```python
from build123d import *

# Parameters (mm, degrees)
F0_R             = 21
F1_DEPTH         = 7
F3_DEPTH         = 3
F4_R             = 3.35
F5_DEPTH         = 2
F6_R             = 0.5
F7_DEPTH         = 3.4
F8_R             = 5
F9_DEPTH         = 5.5
F13_COPIES_COUNT = 4


# Not quite as in the source:
# - a pattern or mirror of a feature is missing from the dataset's text; its kind, count and spacing are read off the source's solid


with BuildPart() as f1:
    # F0 (on Top) → F1 (new body)
    with BuildSketch(Plane.XY):
        Circle(F0_R)
    extrude(amount=F1_DEPTH)

    # F2 (on face) → F3 (cut)
    with BuildSketch(Plane.XY.offset(7)):
        with BuildLine():
            Line((-2.5, 16.8585155142), (-4.3, 4.4317744753))
            ThreePointArc((-4.3, 4.4317744753), (-6.175, 0), (-4.3, -4.4317744753))
            Line((-4.3, -4.4317744753), (-2.5, -16.8585155142))
            ThreePointArc((-2.5, -16.8585155142), (-1.6521982913, -18.3987898667), (0, -19))
            ThreePointArc((0, -19), (1.6521982913, -18.3987898667), (2.5, -16.8585155142))
            Line((2.5, -16.8585155142), (4.3, -4.4317744753))
            ThreePointArc((4.3, -4.4317744753), (6.175, 0), (4.3, 4.4317744753))
            Line((4.3, 4.4317744753), (2.5, 16.8585155142))
            ThreePointArc((2.5, 16.8585155142), (1.6521982913, 18.3987898667), (0, 19))
            ThreePointArc((0, 19), (-1.6521982913, 18.3987898667), (-2.5, 16.8585155142))
        make_face()
    extrude(amount=-F3_DEPTH, mode=Mode.SUBTRACT)

    # F4 (on face) → F5 (cut)
    with BuildSketch(Plane.XY.offset(4)):
        Circle(F4_R)
    extrude(amount=-F5_DEPTH, mode=Mode.SUBTRACT)

    # F6 (on face) → F7 (cut)
    with BuildSketch(Plane.XY.offset(4)):
        with Locations((0, 7.375)):
            Circle(F6_R)
        with Locations((0, 10.375)):
            Circle(F6_R)
        with Locations((0, 13.375)):
            Circle(F6_R)
        with Locations((0, 16.375)):
            Circle(F6_R)
        with Locations((0, -7.375)):
            Circle(F6_R)
        with Locations((0, -10.375)):
            Circle(F6_R)
        with Locations((0, -13.375)):
            Circle(F6_R)
        with Locations((0, -16.375)):
            Circle(F6_R)
    extrude(amount=-F7_DEPTH, mode=Mode.SUBTRACT)

    # F8 (on face) → F9 (cut, through all)
    with BuildSketch(Plane.XY.offset(7)):
        with Locations((-12, 0)):
            Circle(F8_R)
        with Locations((12, 0)):
            Circle(F8_R)
    extrude(amount=-F9_DEPTH, mode=Mode.SUBTRACT)

    # F12 (on plane+point) → F13 (revolve, cut)
    with BuildSketch(Plane.XZ.offset(10.6066017178)):
        with BuildLine():
            Line((-10.6066017178, 0), (-10.6066017178, 7))
            Line((-10.6066017178, 7), (-11.6066017178, 7.0008294335))
            Line((-11.6066017178, 7.0008294335), (-11.6066017178, 4.2948370387))
            ThreePointArc((-11.6066017178, 4.2948370387), (-13.8675802694, 0.6440169112), (-10.6066017178, -2.15))
            Line((-10.6066017178, -2.15), (-10.6066017178, 0))
        make_face()
    f13 = revolve(axis=Axis((-10.6066017178, -10.6066017178, -1.075), (0, 0, -1)), mode=Mode.SUBTRACT)

    # F13_copies: F13 ×4 about axis
    f13_copies_axis = Axis((0, 0, 0), (0, 0, 1))
    for i in range(1, F13_COPIES_COUNT):
        add(f13.rotate(f13_copies_axis, i * 360 / F13_COPIES_COUNT), mode=Mode.SUBTRACT)


solid = f1.part
```
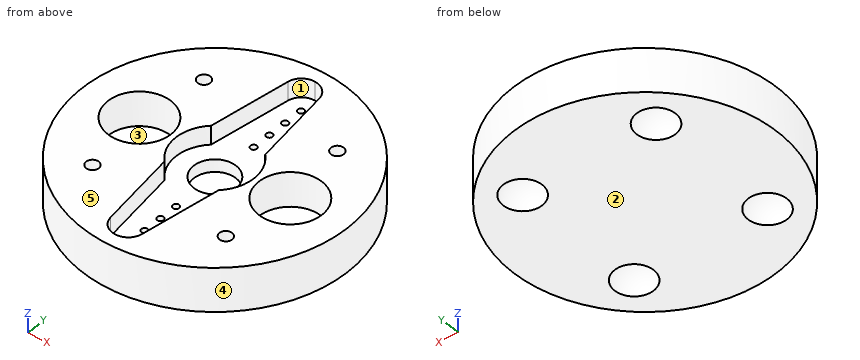
Read the model definition and answer for the solid it produces. Units are mm, in the model's axes. Face numbers are marked on the shaded views. A direction names the side the tool comes from. Coordinates: 2 decimals unless noted, no trailing zeros. Write each loop counter-clockwise with the first axis right and the second up, starting at its lowest first coordinate (ties: lowest second). Pieces come first, ordered by that corner, then holes. Notation, with made-up numbers: (85, 58.5) -> (110, 58.5) arc R14 cw to (110, 65.5) -> close; hole circle Ø10 at (56.5, -14.75). An arc over 180 degrees is marked (long way). Write item = value, one per line.
(1) Section B-B on z = 2.5 is taken. Count the separate pieces of the cut face and the enclosed holes in it, plus the area to 3 significant figures.
From the geometry:
separate_pieces = 1
enclosed_holes = 15
area = 1,070 mm2
(2) Section D-D on y = -15 is taken. Write down the section's boundary in (x, z), plus the area to 3 significant figures.
From the geometry:
outline = (-14.7, 0) -> (14.7, 0) -> (14.7, 7) -> (2.77, 7) -> (2.77, 4) -> (-2.77, 4) -> (-2.77, 7) -> (-14.7, 7) -> close
area = 189 mm2
(3) Section A-A on y = 0 is taken. Write down the section's boundary in (x, z) (3 decimals), plus the area to 3 significant figures.
From the geometry:
outline = (-21, 0) -> (21, 0) -> (21, 7) -> (17, 7) -> (17, 1.5) -> (7, 1.5) -> (7, 7) -> (6.175, 7) -> (6.175, 4) -> (3.35, 4) -> (3.35, 2) -> (-3.35, 2) -> (-3.35, 4) -> (-6.175, 4) -> (-6.175, 7) -> (-7, 7) -> (-7, 1.5) -> (-17, 1.5) -> (-17, 7) -> (-21, 7) -> close
area = 134 mm2
(4) Which of the six approach directions +Z, -Z, +X, -X, +Y, -Y give full straight-line access (tool end or side, diameter ignored) to the marked faces 1 and 2?
From the geometry:
face_1 = +Z
face_2 = -Z, +X, -X, +Y, -Y
(5) For a pull along Y with two mould halves and no side action, classify the marked faces 3, 4 and 5 as +Y half, -Y half, draft (parallel to the pull), parting line (faces both ways), or undercut.
From the geometry:
face_3 = undercut
face_4 = parting line
face_5 = draft
(6) Given pin 1 Ø2 at (y, z) = (-14.5, 5) entering from -X; pin 2 Ø0.5 at (x, y) = (0, -16) entering from +Z; pin 3 Ø4 at (y, z) = (5, 3) entering from +X, each flat-ended and moving along its own axis, determine where each tip first touches the part or whether it passes through.
From the geometry:
pin_1 = -16.09
pin_2 = 4
pin_3 = 20.78
(7) Straight lines are drawn through the part: L1, parallel to X at y = 3.5, z = 2.5; L2, parallel to X at y = 1, z = 3.5; L3, parallel to Y at x = 9, z = 1. For each, find the intervals that lie inside material, in ascending order. Write a range as from..to.
From the geometry:
L1 = -20.71..-15.57, -8.43..8.43, 15.57..20.71
L2 = -20.98..-16.9, -7.1..-3.2, 3.2..7.1, 16.9..20.98
L3 = -18.97..-13.49, -7.73..7.73, 13.49..18.97
(8) Section C-C on x = 2 is taken. Write down the section's boundary in (y, z).
From the geometry:
outline = (-20.9, 0) -> (20.9, 0) -> (20.9, 7) -> (18.03, 7) -> (18.03, 4) -> (2.69, 4) -> (2.69, 2) -> (-2.69, 2) -> (-2.69, 4) -> (-18.03, 4) -> (-18.03, 7) -> (-20.9, 7) -> close
